The model under review builds one solid part; all positions refer to its coordinate system, in mm. A direction names the side the tool comes from. Coordinates: 2 decimals unless noted, no trailing zeros. Order: outer loops, then holes, each group sorted by start corner. A loop starts at its lowest first (then second) coordinate and runs counter-clockwise, first axis right, second up. Notation, with made-up numbers: (70.25, 75.5) - (105.25, 75.5) arc R20 ccw to (105.25, 100.5) - close; hole circle Ø4 at (25.5, 85). An arc over 180 degrees is marked (long way). Answer in a Markdown table with one row per item.
Autodesk Inventor part; units mm, degrees
ref_plane "YZ Plane" through (0, 0, 0) normal (1, 0, 0) x (0, 1, 0)
ref_plane "XZ Plane" through (0, 0, 0) normal (0, 1, 0) x (-1, 0, 0)
ref_plane "XY Plane" through (0, 0, 0) normal (0, 0, 1) x (1, 0, 0)
sketch "スケッチ1" plane through (0, 0, 0) normal (0, 0, 1) x (1, 0, 0)
  circle A0 centre (0, 0) radius 12
  dimension "HUB_DIA" = 24
extrude "ハブ" add sketch "スケッチ1" along normal blind 2
sketch "スケッチ2" plane through (0, 0, 0) normal (0, 0, 1) x (1, 0, 0)
  circle A0 centre (0, 0) radius 22.5
  circle A1 centre (0, 0) radius 21.3
  dimension "DIA" = 45
  dimension "RIM_THIN" = 1.2
extrude "リム" add sketch "スケッチ2" along normal blind 10
sketch "スケッチ5" plane through (0, 0, 0) normal (1, 0, 0) x (0, 1, 0)
  line L0 (21.3, 10) -> (21.3, 0)
  line L1 (21.3, 10) -> (21.3, 0)
  line L2 (21.3, 0) -> (11.5, 0)
  line L3 (22.5, 0) -> (-22.5, 0)
  line L4 (11.5, 0) -> (11.5, 2)
  line L5 (11.5, 2) -> (21.3, 10)
  line L6 (12, 2) -> (-12, 2)
  point P0 (0, 0)
  point P1 (0, 0)
  dimension "d10" = 11.5
extrude "スポーク" add sketch "スケッチ5" along normal mid plane 2
pattern_circular "円形状パターン1" count 4 over 360 about axis through (0, 0, -10) along (0, 0, 1) of "スポーク"
sketch "スケッチ6" plane through (0, 0, 2) normal (0, 0, 1) x (1, 0, 0)
  circle A0 centre (0, 0) radius 8 construction
  line L0 (-13.4189, -13.4189) -> (13.4189, 13.4189) construction
  line L1 (-15.0493, 15.0493) -> (15.0493, -15.0493) construction
  line L2 (-16.6434, 0) -> (16.6434, 0) construction
  point P0 (5.6569, 5.6569)
  point P1 (-5.6569, 5.6569)
  point P2 (-5.6569, -5.6569)
  point P3 (5.6569, -5.6569)
  dimension "d16" = 16
  dimension "d17" = 45
  dimension "d18" = 45
hole "フランジ取付穴" at (5.6569, 5.6569, 2) at (-5.6569, 5.6569, 2) at (-5.6569, -5.6569, 2) at (5.6569, -5.6569, 2) direction (0, 0, -1) diameter 3.2 end through all
sketch "スケッチ8" plane through (0, 0, 0) normal (0, 0, -1) x (-1, 0, 0)
  circle A0 centre (5.6569, 5.6569) radius 1.6 construction
  line L0 (5.6569, 5.6569) -> (10.4286, 10.4286) construction
  line L1 (5.6569, 5.6569) -> (12.4051, 5.6569) construction
  line L2 (5.7276, 5.5861) -> (5.5861, 5.7276)
  line L3 (5.5861, 5.7276) -> (11.243, 11.3844)
  line L4 (11.243, 11.3844) -> (11.3844, 11.243)
  line L5 (11.3844, 11.243) -> (5.7276, 5.5861)
  point P0 (0, 0)
  dimension "d32" = 45
  dimension "d33" = 8
  dimension "d34" = 0.2
extrude "1層目をきれいに出力する溝" cut sketch "スケッチ8" against normal blind 0.2
pattern_circular "円形状パターン2" count 4 over 360 about axis through (0, 0, -10) along (0, 0, 1) of "1層目をきれいに出力する溝"
equation "\"d18\" = d17"
properties part number "Wheel-D45A"
Item 1: We need section D-D, the plane z = 5.75. Write out the cut boundary in (x, y), then the cut area to 3 significant figures.
Check values:
| item | result |
|---|---|
| outline | circle Ø45 at (0, 0); hole (-21.28, -1) arc R21.3 ccw to (-1, -21.28) - (-1, -16.09) - (1, -16.09) - (1, -21.28) arc R21.3 ccw to (21.28, -1) - (16.09, -1) - (16.09, 1) - (21.28, 1) arc R21.3 ccw to (1, 21.28) - (1, 16.09) - (-1, 16.09) - (-1, 21.28) arc R21.3 ccw to (-21.28, 1) - (-16.09, 1) - (-16.09, -1) - close |
| area | 207 mm^2 |
Item 2: Tool access review of faces 4 (the face through (16.331, 0.014, 5.944)), 5 (the face through (-8.4, -8.57, 0.99)): name each direction out of +Z, -Z, +X, -X, +Y, -Y from which nothing blocks a thin tool from reaching the whole face with its end or side.
Check values:
| item | result |
|---|---|
| face 4 | +Z |
| face 5 | +Z, -Z |
Item 3: We need section A-A, the plane x = 15. Write out the cut boundary in (y, z).
Check values:
| item | result |
|---|---|
| outline | (-16.77, 0) - (-15.12, 0) - (-15.12, 10) - (-16.77, 10) - close; (-1, 0) - (1, 0) - (1, 4.86) - (-1, 4.86) - close; (15.12, 0) - (16.77, 0) - (16.77, 10) - (15.12, 10) - close |
Item 4: Clearance check with flat-ended pins moving along their axes: pin 1 Ø5 at (x, z) = (-2.5, 6.5) entering from -Y; pin 2 Ø1 at (y, z) = (-17, 4.5) entering from +X; pin 3 Ø4 at (x, z) = (-7, 2.5) entering from -Y. State where each tip first meets the part, or that it passes through.
Check values:
| item | result |
|---|---|
| pin 1 | y = -22.5 |
| pin 2 | x = 15.3 |
| pin 3 | y = -21.94 |
Item 5: We need section B-B, the plane y = 19. Write out the cut boundary in (x, z), then the cut area to 3 significant figures.
Check values:
| item | result |
|---|---|
| outline | (-12.05, 0) - (-9.63, 0) - (-9.63, 10) - (-12.05, 10) - close; (-1, 0) - (1, 0) - (1, 8.12) - (-1, 8.12) - close; (9.63, 0) - (12.05, 0) - (12.05, 10) - (9.63, 10) - close |
| area | 64.7 mm^2 |
Item 6: Mouldability with a two-part tool opening along X and no side actions: class faces 1 (the face through (8, -20, 10)), 2 (the face through (15.23, -14.89, 4.93)), 3 (the face through (4.308, 4.797, 0.986)) as +X half, -X half, draft (parallel to the pull), parting line (faces both ways), or undercut.
Check values:
| item | result |
|---|---|
| face 1 | draft |
| face 2 | undercut |
| face 3 | undercut |
Item 7: To check wall thickness, follow line 1 (Y direction, x = 16, z = 3); line 2 (Y direction, x = 15.5, z = 2); line 3 (X direction, y = 18.5, z = 5.25). State the ranges of each line that lie inside material, in increasing order. Write a range as from..to.
Check values:
| item | result |
|---|---|
| line 1 | -15.82..-14.06, -1..1, 14.06..15.82 |
| line 2 | -16.31..-14.61, -1..1, 14.61..16.31 |
| line 3 | -12.81..-10.56, -1..1, 10.56..12.81 |
Item 8: We need section C-C, the plane z = 8.75. Write out the cut boundary in (x, y), then the cut area to 3 significant figures.
Check values:
| item | result |
|---|---|
| outline | circle Ø45 at (0, 0); hole (-21.28, -1) arc R21.3 ccw to (-1, -21.28) - (-1, -19.77) - (1, -19.77) - (1, -21.28) arc R21.3 ccw to (21.28, -1) - (19.77, -1) - (19.77, 1) - (21.28, 1) arc R21.3 ccw to (1, 21.28) - (1, 19.77) - (-1, 19.77) - (-1, 21.28) arc R21.3 ccw to (-21.28, 1) - (-19.77, 1) - (-19.77, -1) - close |
| area | 177 mm^2 |
